Geometry: final body of the model. Coordinates: model frame, mm. A direction names the side the tool comes from. Give positions to 0.01 mm unless a question says otherwise; leave off trailing zeros. Loops run counter-clockwise (first coordinate to the right, second up) from the corner with the lowest first, then second, coordinate; pieces in that order, holes last.
1. First-contact query: P1, Ø1, axis at y = 3, z = 59.5, coming from the -X side; P2, Ø1.5, axis at y = -8.5, z = 18, coming from the +X side; P3, Ø8, axis at x = 18, z = 67, coming from the +Y side. Flat tips, straight axial feed; report the tip coordinate or a pass-through.
2. Section C-C, the plane z = 37.5. Output: boundary loops of the cut face in (x, y).
3. Draft query along Y for faces 1 (the face through (-22.448, -15.236, 38.633)), 2 (the face through (-30.235, -23.183, 37.656)), 3 (the face through (28, 2, 76.2)). Return one class per face: +Y half, -Y half, draft (parallel to the pull), parting line (faces both ways), or undercut.
4. Section A-A, the plane z = 23. Output: boundary loops of the cut face in (x, y).
5. Material intervals for line 1 along X through (y, z) = (12.5, 64.5); line 2 along Y through (x, z) = (-10.5, 68.5); line 3 along Y through (x, z) = (-21, 53), sorted ascending.
6. Section B-B, the plane x = 0. Output: boundary loops of the cut face in (y, z).
7. Access query for faces 4 (the face through (-30.4, 8.5, 76.2)), 5 (the face through (-1.878, -26.607, 38.633)). Directions: +Z, -Z, +X, -X, +Y, -Y. A direction counts if a zero-diameter tool reaches every point of the face in a straight line with its end or side. Return the directions, or none.
from build123d import *

# Parameters (mm, degrees)
F0_R     = 38.1
F1_DEPTH = 76.2
F3_DEPTH = 76.2
F4_R     = 6.35
F5_DEPTH = 3.81
F6_DEPTH = 6.35
F7_R     = 6.35
F8_DEPTH = 12.7


# Not quite as in the source:
# - the program builds the solid bodies; features that only make, move or delete a surface that nothing else refers to are left out


with BuildPart() as f1:
    # F0 (on Top) → F1 (new body)
    with BuildSketch(Plane.XY):
        Circle(F0_R)
    extrude(amount=F1_DEPTH)

    # F2 (on face) → F3 (cut)
    with BuildSketch(Plane.XY.offset(76.2)):
        Polygon((-22.9046876713, 20.3177796807), (-29.9596701578, -4.7970021274), (-14.7228526975, -25.9716198769), (11.3321303875, -27.2611545189), (28.5853454095, -7.6945601662), (24.0447695554, 17.9941185477), (1.1295490542, 30.4607825978), align=None)
    extrude(amount=-F3_DEPTH, mode=Mode.SUBTRACT)

    # F4
    f4_edges = [f1.edges().sort_by_distance(p)[0] for p in [
        (38.1, 0, 38.1),
        (-38.1, 0, 0),
        (-38.1, 0, 76.2),
    ]]
    fillet(f4_edges, radius=F4_R)

    # F5 (cut): a face of the model
    f5_faces = [f1.faces().sort_by_distance(p)[0] for p in [
        (-26.4321789145, 7.7603887767, 38.1),
    ]]
    extrude(f5_faces, amount=-F5_DEPTH, mode=Mode.SUBTRACT)

    # F6 (add): a face of the model
    f6_faces = [f1.faces().sort_by_distance(p)[0] for p in [
        (-24.7355489473, 20.8320861293, 38.1),
    ]]
    extrude(f6_faces, amount=F6_DEPTH)

    # F7 (on face) → F8 (cut)
    with BuildSketch(Plane(origin=(-30.1875139729, 8.4799614831, 0), x_dir=(0.2704418413, 0.9627363141, 0), z_dir=(0.9627363141, -0.2704418413, 0))):
        with Locations((-2.3566866294, 41.5975786746)):
            Circle(F7_R)
    extrude(amount=-F8_DEPTH, mode=Mode.SUBTRACT)


solid = f1.part
Answers below:
1. P1: stops at x = -38.02
1. P2: stops at x = 37.3
1. P3: stops at y = 35.43
2. outline: (-37.97, 3.18) arc R38.1 ccw (long way) to (-35.93, 12.68) - (-29.51, 10.88) - (-28.29, 15.23) - (-24.62, 14.2) - (-22.9, 20.32) - (1.13, 30.46) - (24.04, 17.99) - (28.59, -7.69) - (11.33, -27.26) - (-14.72, -25.97) - (-29.96, -4.8) - (-33.63, -3.77) - (-32.14, 1.54) - close
3. face 1: undercut
3. face 2: parting line
3. face 3: draft
4. outline: circle Ø76.2 at (0, 0); hole (-33.63, -3.77) - (-29.96, -4.8) - (-14.72, -25.97) - (11.33, -27.26) - (28.59, -7.69) - (24.04, 17.99) - (1.13, 30.46) - (-22.9, 20.32) - (-24.62, 14.2) - (-28.29, 15.23) - close
5. line 1: x = -35.99 to -29.06, 25.02 to 35.99
5. line 2: y = -36.62 to -26.18, 25.55 to 36.62
5. line 3: y = -31.79 to -17.25, 21.12 to 31.79
6. outline: (-38.1, 6.35) arc R6.35 ccw to (-31.75, 0) - (-26.7, 0) - (-26.7, 76.2) - (-31.75, 76.2) arc R6.35 ccw to (-38.1, 69.85) - close; (29.98, 0) - (31.75, 0) arc R6.35 ccw to (38.1, 6.35) - (38.1, 69.85) arc R6.35 ccw to (31.75, 76.2) - (29.98, 76.2) - close
7. face 4: +Z, +X, -X, +Y, -Y
7. face 5: +Z, -Z
